Source: CAD feature listing. Evaluate the final solid. Frame: model axes, mm. A direction names the side the tool comes from. Round coordinates to 2 decimals unless told otherwise and drop trailing zeros. Write each loop counter-clockwise with the first axis right and the second up, starting at its lowest first coordinate (ties: lowest second). Pieces come first, ordered by that corner, then holes.
```python
from build123d import *

# Parameters (mm, degrees)
F0_W     = 130
F0_H     = 150
F1_DEPTH = 110
F2_R     = 37.5
F3_DEPTH = 130
F5_DEPTH = 100
F6_DEPTH = 1


with BuildPart() as f1:
    # F0 (on Front) → F1 (new body)
    with BuildSketch(Plane.XZ):
        Rectangle(F0_W, F0_H)
    extrude(amount=-F1_DEPTH)

    # F2 (on face) → F3 (cut)
    with BuildSketch(Plane.YZ.offset(65)):
        with Locations((55, 0)):
            Circle(F2_R)
    extrude(amount=-F3_DEPTH, mode=Mode.SUBTRACT)

    # F4 (on Front) → F5 (join)
    with BuildSketch(Plane.XZ):
        Polygon((-9, 0), (9, 0), (0, 17.860571), align=None)
    extrude(amount=F5_DEPTH)

    # F4 (on Front) → F6 (join)
    with BuildSketch(Plane.XZ):
        Polygon((-44.622627, 34.545667), (-24.622664, 34.507253), (-34.589379, 51.846936), align=None)
        Polygon((21.962458, 34.184783), (41.962421, 34.14637), (31.995706, 51.486053), align=None)
    extrude(amount=F6_DEPTH)


solid = f1.part
```
Q1. Section query B-B, the plane x = 45.5. Output: boundary loops of the cut face in (y, z), and give its area (3 significant figures).
Q2. Set-up query: faces 1 (the face through (0, -49, 0)), 2 (the face through (32, -1, 41)), 3 (the face through (-39.536, -0.493, 43.317)), 4 (the face through (37.05, -0.49, 42.69)). Return all of +Z, -Z, +X, -X, +Y, -Y with unobstructed straight access to the full face (end or side cutting, diameter ignored); none if empty.
Q3. Pin query (flat end, axial travel): P1, Ø1.5, axis at x = -2.5, y = -20, coming from the -Z side; P2, Ø6, axis at x = 10, z = -35.5, coming from the -Y side; P3, Ø8.5, axis at x = -32, z = 46, coming from the -Y side. Return the tip coordinate at first contact, or that it passes through.
Q4. Section query A-A, the plane y = 55. Output: boundary loops of the cut face in (x, z).
Q5. Section query C-C, the plane z = 48. Output: boundary loops of the cut face in (x, y), and give its area (3 significant figures).
Q6. Mould query, pull axis X, two halves, no side actions, for faces 5 (the face through (-29.54, -0.49, 43.06)), 6 (the face through (27.05, -0.49, 42.96)), 7 (the face through (-4.437, -49.3, 9.055)), 8 (the face through (-1, 54, 75)). Classes: pulls with the +X half, pulls with the -X half, needs draft (parallel to the pull), parting line crosses it, or undercut.
Q7. Section query D-D, the plane y = -52.5. Output: boundary loops of the cut face in (x, z), and give its area (3 significant figures).
Q8. Line query: line 1 (Z direction, x = -3.5, y = 55); line 2 (Y direction, x = 36, z = -2); line 3 (Z direction, x = -36, y = 74). Output: solid intervals per line, ascending.
Filled in:
1. outline: (0, -75) - (110, -75) - (110, 75) - (0, 75) - close; hole circle Ø75 at (55, 0)
1. area: 12,100 mm2
2. face 1: -Z, +X, -X, -Y
2. face 2: +Z, -Z, +X, -X, -Y
2. face 3: +Z, -X, -Y
2. face 4: +Z, +X, -Y
3. P1: stops at z = 0
3. P2: stops at y = 0
3. P3: stops at y = -1
4. outline: (-65, -75) - (65, -75) - (65, -37.5) - (-65, -37.5) - close; (-65, 37.5) - (65, 37.5) - (65, 75) - (-65, 75) - close
5. outline: (-65, 0) - (-36.82, 0) - (-36.82, -1) - (-32.38, -1) - (-32.38, 0) - (29.97, 0) - (29.97, -1) - (34, -1) - (34, 0) - (65, 0) - (65, 110) - (-65, 110) - close
5. area: 14,300 mm2
6. face 5: undercut
6. face 6: undercut
6. face 7: pulls with the -X half
6. face 8: needs draft
7. outline: (-9, 0) - (9, 0) - (0, 17.86) - close
7. area: 161 mm2
8. line 1: z = -75 to -37.5, 37.5 to 75
8. line 2: y = 0 to 17.55, 92.45 to 110
8. line 3: z = -75 to -32.33, 32.33 to 75
